```python
from build123d import *

# Parameters (mm, degrees)
F0_R          = 1.5875
F1_DEPTH      = 19.05
F2_W          = 6.35
F2_H          = 21.8940776977
F3_DEPTH      = 69.31141
F3_DEPTH_BACK = 25.4
F5_W          = 31.5987952054
F5_H          = 9.1577427173
F6_DEPTH      = 33.02


with BuildPart() as f1:
    # F0 (on Front) → F1 (new body)
    with BuildSketch(Plane.XZ):
        with BuildLine():
            ThreePointArc((3.2306237647, 27.0146857947), (-15.7693382353, 8.0147237947), (-34.7693002353, 27.0146857947))
            Line((-34.7693002353, 27.0146857947), (-44.3443382353, 27.0146857947))
            ThreePointArc((-44.3443382353, 27.0146857947), (-43.9176321109, 31.9344598635), (-42.6502576132, 36.7073014581))
            ThreePointArc((-42.6502576132, 36.7073014581), (-54.1838863729, 27.0146857947), (-42.6502576132, 17.3220701313))
            ThreePointArc((-42.6502576132, 17.3220701313), (-15.5884947503, -1.5597419447), (11.2321092838, 17.6630839601))
            ThreePointArc((11.2321092838, 17.6630839601), (22.288726896, 27.0146857947), (11.2321092838, 36.3662876293))
            ThreePointArc((11.2321092838, 36.3662876293), (12.4095278514, 31.7562183603), (12.8056617647, 27.0146857947))
            Line((12.8056617647, 27.0146857947), (3.2306237647, 27.0146857947))
        make_face()
        with Locations((-48.6005805433, 27.0146857947)):
            Circle(F0_R, mode=Mode.SUBTRACT)
        with Locations((17.8374499083, 27.0146857947)):
            Circle(F0_R, mode=Mode.SUBTRACT)
    extrude(amount=F1_DEPTH)

    # F2 (on Right) → F3 (cut, two sides)
    with BuildSketch(Plane.YZ) as f3_sk:
        with Locations((-9.525, 27.4422825678)):
            Rectangle(F2_W, F2_H)
    extrude(amount=-F3_DEPTH, mode=Mode.SUBTRACT)
    extrude(f3_sk.sketch, amount=F3_DEPTH_BACK, mode=Mode.SUBTRACT)

    # F5 (on plane+point) → F6 (cut)
    with BuildSketch(Plane.XY.offset(36.7073014581)):
        with Locations((-15.7993976027, -13.0069836187)):
            Rectangle(F5_W, F5_H)
    extrude(amount=-F6_DEPTH, mode=Mode.SUBTRACT)


solid = f1.part
```
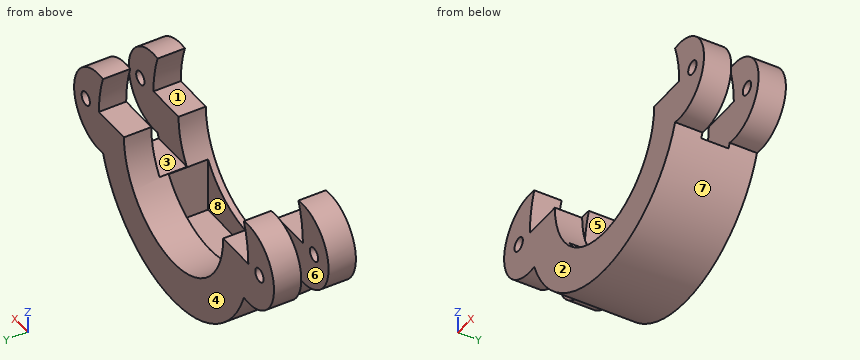
Source: CAD feature listing. Evaluate the final solid. Frame: model axes, mm. Face numbers are marked on the shaded views. A direction names the side the tool comes from. Round coordinates to 2 decimals unless told otherwise and drop trailing zeros. Order: outer loops, then holes, each group sorted by start corner. A loop starts at its lowest first (then second) coordinate and runs counter-clockwise, first axis right, second up. Notation, with made-up numbers: (61, -35.5) -> (100, -35.5) arc R20 ccw to (100, -23.5) -> close; hole circle Ø5 at (10, 80.5). An arc over 180 degrees is marked (long way). One line per item, written item: value. Start each with the question number.
Q1. Material intervals for probe 1 along Y at (x, z) = (-23.5, 8.5); probe 2 along Y at (x, z) = (8.5, 23); probe 3 along Z at (x, y) = (17, -13), sorted ascending.
Q2. Access query for the marked faces 4, 5, 6, 7 and 8. Directions: +Z, -Z, +X, -X, +Y, -Y. A direction counts if a zero-diameter tool reaches every point of the face in a straight line with its end or side. Return the directions, or none.
Q3. Draft query along Z for the marked faces 1, 2 and 3. Return one class per face: pulls with the +Z half, pulls with the -Z half, needs draft (parallel to the pull), parting line crosses it, or undercut.
Q4. Section query D-D (x = -2). Return the cut outline in (y, z).
Q5. Section query C-C (y = -11.5). Return the cut outline in (x, z) (3 decimals), plus the area to 3 significant figures.
Q6. Section query A-A (z = 11). Return the cut outline in (x, y), plus the area to 3 significant figures.
Q7. Section query B-B (z = 22.5). Return the cut outline in (x, y).
Q8. Pin query (flat end, axial travel): pin 1 (7 mm diameter, centred on x = -40, y = -16, fed in from +Z); pin 2 (5 mm diameter, centred on x = -43.5, y = -12, fed in from -Z); pin 3 (6 mm diameter, centred on x = -5.5, z = 3, fed in from +Y); pin 4 (1.5 mm diameter, centred on x = 8.5, y = -12.5, fed in from -Z). Return the tip coordinate at first contact, or that it passes through.
Findings below:
1. probe 1: -19.05 to -17.59, -8.43 to 0
1. probe 2: -19.05 to -12.7, -6.35 to 0
1. probe 3: 18.51 to 25.67, 28.36 to 35.52
2. face 4: +Z, -Z, +X, -X, +Y
2. face 5: +Y, -Y
2. face 6: +Z, +X, -X
2. face 7: -Z, +Y, -Y
2. face 8: +Z
3. face 1: undercut
3. face 2: needs draft
3. face 3: pulls with the +Z half
4. outline: (-19.05, 1.98) -> (0, 1.98) -> (0, 13.92) -> (-8.43, 13.92) -> (-8.43, 3.69) -> (-17.59, 3.69) -> (-17.59, 13.92) -> (-19.05, 13.92) -> close
5. outline: (-42.338, 16.495) arc R28.575 ccw to (10.799, 16.495) -> (0.053, 16.495) arc R19 cw to (0, 16.416) -> (0, 3.687) -> (-31.599, 3.687) -> (-31.599, 16.495) -> close
5. area: 291 mm²
6. outline: (-39.43, -19.05) -> (-25.99, -19.05) -> (-25.99, -17.59) -> (-31.6, -17.59) -> (-31.6, -8.43) -> (-25.99, -8.43) -> (-25.99, 0) -> (-39.43, 0) -> close; (-5.55, -19.05) -> (7.9, -19.05) -> (7.9, 0) -> (-5.55, 0) -> (-5.55, -8.43) -> (0, -8.43) -> (0, -17.59) -> (-5.55, -17.59) -> close
6. area: 410 mm²
7. outline: (-53.09, -19.05) -> (-34.23, -19.05) -> (-34.23, -12.7) -> (-53.09, -12.7) -> close; (-53.09, -6.35) -> (-34.23, -6.35) -> (-34.23, 0) -> (-53.09, 0) -> close; (2.69, -19.05) -> (21.15, -19.05) -> (21.15, -12.7) -> (2.69, -12.7) -> close; (2.69, -6.35) -> (21.15, -6.35) -> (21.15, 0) -> (2.69, 0) -> close
8. pin 1: z = 36.82
8. pin 2: z = 13.6
8. pin 3: y = 0
8. pin 4: z = 10.79
